Source: CAD feature listing. Evaluate the final solid. Frame: model axes, mm. Face numbers are marked on the shaded views. A direction names the side the tool comes from. Coordinates: 2 decimals unless noted, no trailing zeros. Write each loop counter-clockwise with the first axis right and the second up, starting at its lowest first coordinate (ties: lowest second). Pieces come first, ordered by that corner, then holes. Notation, with made-up numbers: (63.25, 17) - (71.25, 17) arc R29 cw to (71.25, 44) - close; hole circle Ø10 at (-22.75, 18.5). An arc over 180 degrees is marked (long way). One line per question, with ' | ' between items. Start each with the question number.
Q1. Cut plane C-C, the plane y = -18.5. Return loops of the section in (x, z).
Q2. Contact query for flat-ended pins moving along their axis: P1, Ø10, axis at x = -37.5, z = 30, coming from the -Y side; P2, Ø1.5, axis at y = 14.5, z = 25, coming from the -X side; P3, Ø2, axis at x = -30.5, y = 24.5, coming from the -Z side; P4, Ø1.8, axis at x = -33.5, z = 41.5, coming from the -Y side. Output: stop coordinate, or through.
Q3. Cut plane D-D, the plane x = -31.5. Return loops of the section in (y, z).
Q4. Cut plane A-A, the plane y = -8.5. Return loops of the section in (x, z), plus the area to 3 significant figures.
Q5. Line query: line 1 (Z direction, x = -35.5, y = 3.5); line 2 (Y direction, x = -44.5, z = 21); line 3 (Z direction, x = -32, y = 22). Output: solid intervals per line, ascending.
Q6. Cut plane B-B, the plane x = -37. Return loops of the section in (y, z).
Q7. Access query for the marked faces 4, 5 and 6. Directions: +Z, -Z, +X, -X, +Y, -Y. A direction counts if a zero-diameter tool reaches every point of the face in a straight line with its end or side. Return the directions, or none.
Q8. Draft query along X for the marked faces 1, 2 and 3. Return one class per face: +X half, -X half, draft (parallel to the pull), parting line (faces both ways), or undercut.
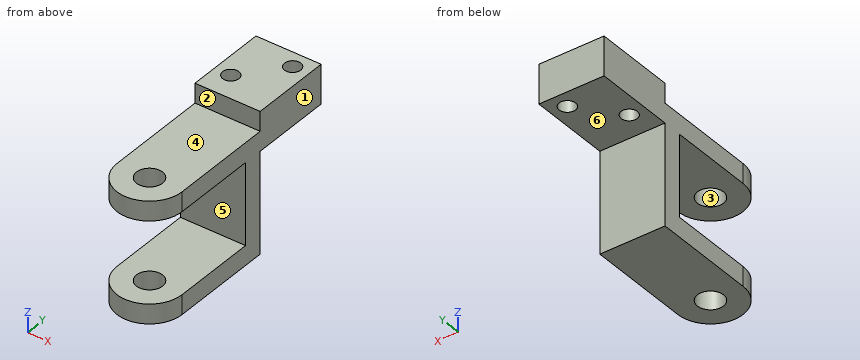
```python
from build123d import *

# Parameters (mm, degrees)
EXTRUDE_1_DEPTH     = 37
SKETCH_5_R          = 4
CUT_EXTRUDE_1_DEPTH = 67.495686501
SKETCH_6_W          = 25
SKETCH_6_H          = 39.826286975
CUT_EXTRUDE_2_DEPTH = 52.661548552
SKETCH_8_W          = 20
SKETCH_8_H          = 25
EXTRUDE_5_DEPTH     = 6
SKETCH_8_3_W        = 20
SKETCH_8_3_H        = 25
EXTRUDE_6_DEPTH     = 6
SKETCH_10_W         = 20
SKETCH_10_H         = 25
EXTRUDE_7_DEPTH     = 6
SKETCH_11_R         = 2.5
CUT_EXTRUDE_3_DEPTH = 67.954199448


with BuildPart() as part:
    # Sketch 1 → Extrude 1 (new body)
    with BuildSketch(Plane.XY):
        with BuildLine():
            Line((-26.397852585, -19.99859328), (-26.397852585, 12.00140672))
            Line((-26.397852585, 12.00140672), (-46.397852585, 12.00140672))
            Line((-46.397852585, 12.00140672), (-46.397852585, -19.99859328))
            ThreePointArc((-46.397852585, -19.99859328), (-36.397852585, -29.99859328), (-26.397852585, -19.99859328))
        make_face()
    extrude(amount=EXTRUDE_1_DEPTH)

    # Sketch 5 → Cut-Extrude 1 (cut, through all)
    with BuildSketch(Plane(origin=(0, 0, 0), x_dir=(-1, 0, 0), z_dir=(0, 0, -1))):
        with Locations((36.397852585, -19.99859328)):
            Circle(SKETCH_5_R)
    extrude(amount=-CUT_EXTRUDE_1_DEPTH, mode=Mode.SUBTRACT)

    # Sketch 6 → Cut-Extrude 2 (cut, through all)
    with BuildSketch(Plane(origin=(-26.397852585, 0, 0), x_dir=(0, 0, -1), z_dir=(1, 0, 0))):
        with Locations((-18.5, -13.911736768)):
            Rectangle(SKETCH_6_W, SKETCH_6_H)
    extrude(amount=-CUT_EXTRUDE_2_DEPTH, mode=Mode.SUBTRACT)



with BuildPart() as body_2:
    # Sketch 8 → Extrude 5 (new body)
    with BuildSketch(Plane.XY.offset(37)):
        with Locations((-36.397852585, 24.50140672)):
            Rectangle(SKETCH_8_W, SKETCH_8_H)
    extrude(amount=EXTRUDE_5_DEPTH)

    # Sketch 8_3 → Extrude 6 (add)
    with BuildSketch(Plane.XY.offset(37)):
        with Locations((-36.397852585, 24.50140672)):
            Rectangle(SKETCH_8_3_W, SKETCH_8_3_H)
    extrude(amount=EXTRUDE_6_DEPTH)


with BuildPart() as part_1:
    add(part.part)

    add(body_2.part)  # Extrude 7 merges body 2
    # Sketch 10 → Extrude 7 (add)
    with BuildSketch(Plane(origin=(0, 0, 37), x_dir=(-1, 0, 0), z_dir=(0, 0, -1))):
        with Locations((36.397852585, 24.50140672)):
            Rectangle(SKETCH_10_W, SKETCH_10_H)
    extrude(amount=EXTRUDE_7_DEPTH)

    # Sketch 11 → Cut-Extrude 3 (cut, through all)
    with BuildSketch(Plane(origin=(0, 0, 31), x_dir=(-1, 0, 0), z_dir=(0, 0, -1))):
        with Locations((31.397852585, 32.00140672)):
            Circle(SKETCH_11_R)
        with Locations((41.397852585, 20.00140672)):
            Circle(SKETCH_11_R)
    extrude(amount=-CUT_EXTRUDE_3_DEPTH, mode=Mode.SUBTRACT)


solid = part_1.part
```
Reply:
1) outline: (-46.4, 0) - (-40.11, 0) - (-40.11, 6) - (-46.4, 6) - close; (-46.4, 31) - (-40.11, 31) - (-40.11, 37) - (-46.4, 37) - close; (-32.69, 0) - (-26.4, 0) - (-26.4, 6) - (-32.69, 6) - close; (-32.69, 31) - (-26.4, 31) - (-26.4, 37) - (-32.69, 37) - close
2) P1: stops at y = -30 | P2: passes through | P3: stops at z = 31 | P4: stops at y = 12
3) outline: (-28.72, 0) - (12, 0) - (12, 31) - (29.5, 31) - (29.5, 43) - (12, 43) - (12, 37) - (-28.72, 37) - (-28.72, 31) - (6, 31) - (6, 6) - (-28.72, 6) - close; (34.5, 31) - (37, 31) - (37, 43) - (34.5, 43) - close
4) outline: (-46.4, 0) - (-26.4, 0) - (-26.4, 6) - (-46.4, 6) - close; (-46.4, 31) - (-26.4, 31) - (-26.4, 37) - (-46.4, 37) - close | area: 240 mm^2
5) line 1: z = 0 to 6, 31 to 37 | line 2: y = 6 to 12 | line 3: z = 31 to 43
6) outline: (-29.98, 0) - (-23.95, 0) - (-23.95, 6) - (-29.98, 6) - close; (-29.98, 31) - (-23.95, 31) - (-23.95, 37) - (-29.98, 37) - close; (-16.04, 0) - (12, 0) - (12, 31) - (37, 31) - (37, 43) - (12, 43) - (12, 37) - (-16.04, 37) - (-16.04, 31) - (6, 31) - (6, 6) - (-16.04, 6) - close
7) face 4: +Z, +X, -X, -Y | face 5: +X, -X, -Y | face 6: -Z, +X, -X, +Y
8) face 1: +X half | face 2: draft | face 3: undercut
